Verification items for the finished model (mm, model axes). Face numbers are marked on the shaded views. A direction names the side the tool comes from. Round coordinates to 2 decimals unless told otherwise and drop trailing zeros. Write each loop counter-clockwise with the first axis right and the second up, starting at its lowest first coordinate (ties: lowest second). Pieces come first, ordered by that corner, then holes. Notation, with made-up numbers: M -4.75,78 L 34.25,78 A20 cw 34.25,85 Z; hole C 42.25,11 d5. An arc over 180 degrees is marked long. One line per item, written item: value. Start each with the question number.
Item 1: Section check B-B, the plane x = 17.5. Record the cut outline in (y, z), then the cut area to 3 significant figures.
Item 2: Thickness scan on probe 1 along X at (y, z) = (2, 35.5); probe 2 along Y at (x, z) = (18.5, 55.5); probe 3 along X at (y, z) = (11.5, 47). Record the ranges inside material, lowest first. Write a range as from..to.
Item 3: Section check D-D, the plane x = 10. Record the cut outline in (y, z).
Item 4: Section check A-A, the plane z = 36. Record the cut outline in (x, y), then the cut area to 3 significant figures.
Item 5: Gauge pin test, flat ends, axial feed: pin 1 (5 mm diameter, centred on x = 17, y = 29, fed in from +Z); pin 2 (1 mm diameter, centred on x = 14.5, z = 41, fed in from -Y). Record the tip position at first contact, or that the pin passes through.
Item 6: Tool access check on the marked faces 5 and 6. Record the directions out of +Z, -Z, +X, -X, +Y, -Y that give a thin tool (end or side, any length) a straight path to the whole face; none if there is none.
Item 7: Section check C-C, the plane y = 12.5. Record the cut outline in (x, z).
Item 8: Draft check along Y on the marked faces 1, 2, 3 and 4. Enter one of: +Y half, -Y half, draft (parallel to the pull), parting line (faces both ways), or undercut.
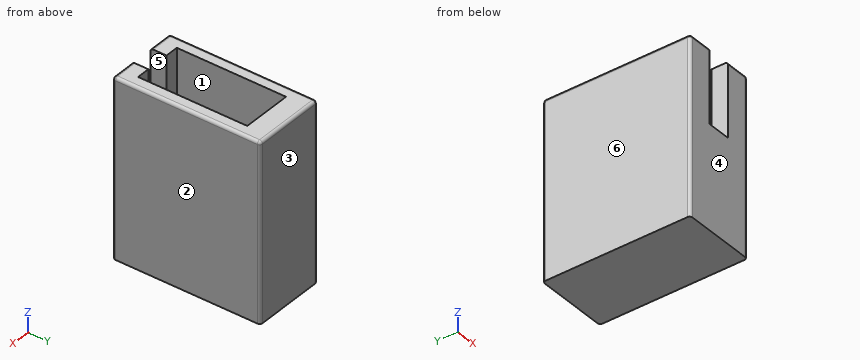
from build123d import *

# Parameters (mm, degrees)
F0_W         = 25
F0_H         = 50
F1_DEPTH     = 60
F2_R         = 1
F4_DEPTH     = 25
F5_T1_DEPTH  = 10
F5_T3_DEPTH  = 10
F5_S7_W      = 1
F5_S7_H      = 1
F5_T8_DEPTH  = 1
F5_S13_W     = 1
F5_S13_H     = 1
F5_T14_DEPTH = 1


# Not quite as in the source:
# - a fillet or chamfer that OpenCascade refuses, or shapes differently, is made with other operations: its cross-section is extruded or revolved along the edge and cut away or added


with BuildPart() as f1:
    # F0 (on Top) → F1 (new body)
    with BuildSketch(Plane.XY):
        with Locations((12.5, 25)):
            Rectangle(F0_W, F0_H)
    extrude(amount=F1_DEPTH)

    # F2
    f2_edges = [f1.edges().sort_by_distance(p)[0] for p in [
        (0, 25, 60),
        (12.5, 50, 60),
        (25, 25, 60),
        (25, 0, 30),
        (0, 0, 30),
        (0, 50, 30),
        (25, 50, 30),
    ]]
    fillet(f2_edges, radius=F2_R)

    # F3 (on face) → F4 (cut)
    with BuildSketch(Plane.XY.offset(60)):
        Polygon((21, 42.5), (4, 42.5), (4, 5.5), (8.5, 5.5), (8.5, 0), (16.5, 0), (16.5, 5.5), (21, 5.5), align=None)
    extrude(amount=-F4_DEPTH, mode=Mode.SUBTRACT)

    # F5: fillet of radius 1 on 2 edges, made by hand

    # F5_s2 → F5_t1 (cut)
    with BuildSketch(Plane.YZ.offset(1)):
        with BuildLine():
            ThreePointArc((0, 59), (0.2928932188, 59.7071067812), (1, 60))
            Line((1, 60), (0, 60))
            Line((0, 60), (0, 59))
        make_face()
    extrude(amount=F5_T1_DEPTH, mode=Mode.SUBTRACT)

    # F5_s4 → F5_t3 (cut)
    with BuildSketch(Plane.YZ.offset(14)):
        with BuildLine():
            ThreePointArc((0, 59), (0.2928932188, 59.7071067812), (1, 60))
            Line((1, 60), (0, 60))
            Line((0, 60), (0, 59))
        make_face()
    extrude(amount=F5_T3_DEPTH, mode=Mode.SUBTRACT)


with BuildPart() as f5_tool6:
    # F5_s7 → F5_t8 (new body)
    with BuildSketch(Plane.XZ.offset(-1)):
        with Locations((24.5, 59.5)):
            Rectangle(F5_S7_W, F5_S7_H)
    extrude(amount=F5_T8_DEPTH)

    # F5_s9 → F5_t10 (revolve, cut)
    with BuildSketch(Plane(origin=(24, 1, 59), x_dir=(-0.7071067812, 0, -0.7071067812), z_dir=(-0.7071067812, 0, 0.7071067812))):
        with BuildLine():
            ThreePointArc((0, -1), (1, 0), (0, 1))
            Line((0, 1), (0, -1))
        make_face()
    revolve(axis=Axis((24, 1, 59), (0, -1, 0)), mode=Mode.SUBTRACT)


with BuildPart() as f1_1:
    add(f1.part)

    # F5_t5: cut F5_tool6
    add(f5_tool6.part, mode=Mode.SUBTRACT)


with BuildPart() as f5_tool12:
    # F5_s13 → F5_t14 (new body)
    with BuildSketch(Plane.XZ.offset(-1)):
        with Locations((0.5, 59.5)):
            Rectangle(F5_S13_W, F5_S13_H)
    extrude(amount=F5_T14_DEPTH)

    # F5_s15 → F5_t16 (revolve, cut)
    with BuildSketch(Plane(origin=(1, 1, 59), x_dir=(0.7071067812, 0, -0.7071067812), z_dir=(-0.7071067812, 0, -0.7071067812))):
        with BuildLine():
            ThreePointArc((0, -1), (1, 0), (0, 1))
            Line((0, 1), (0, -1))
        make_face()
    revolve(axis=Axis((1, 1, 59), (0, -1, 0)), mode=Mode.SUBTRACT)


with BuildPart() as f1_2:
    add(f1_1.part)

    # F5_t11: cut F5_tool12
    add(f5_tool12.part, mode=Mode.SUBTRACT)


solid = f1_2.part
Response values:
1. outline: M 0,0 L 50,0 L 50,59 A1 ccw 49,60 L 42.5,60 L 42.5,35 L 5.5,35 L 5.5,60 L 1,60 A1 ccw 0,59 Z
1. area: 2,070 mm2
2. probe 1: x = 0..8.5, 16.5..25
2. probe 2: y = 0..5.5, 42.5..50
2. probe 3: x = 0..4, 21..25
3. outline: M 0,0 L 50,0 L 50,59 A1 ccw 49,60 L 42.5,60 L 42.5,35 L 0,35 Z
4. outline: M 0,1 A1 ccw 1,0 L 8.5,0 L 8.5,5.5 L 4,5.5 L 4,42.5 L 21,42.5 L 21,5.5 L 16.5,5.5 L 16.5,0 L 24,0 A1 ccw 25,1 L 25,49 A1 ccw 24,50 L 1,50 A1 ccw 0,49 Z
4. area: 576 mm2
5. pin 1: stops at z = 35
5. pin 2: stops at y = 42.5
6. face 5: +Z, -Y
6. face 6: +Z, -Z, -X, +Y, -Y
7. outline: M 0,0 L 25,0 L 25,59 A1 ccw 24,60 L 21,60 L 21,35 L 4,35 L 4,60 L 1,60 A1 ccw 0,59 Z
8. face 1: undercut
8. face 2: draft
8. face 3: +Y half
8. face 4: -Y half
